The listing builds one solid part. Answer for the finished solid, in the listing's coordinates (mm). Face numbers are marked on the shaded views. Round coordinates to 2 decimals unless told otherwise and drop trailing zeros. Write each loop counter-clockwise with the first axis right and the second up, starting at its lowest first coordinate (ties: lowest second). Pieces come first, ordered by that corner, then holes. Notation, with made-up numbers: M 71.5,-16.75 L 103.5,-16.75 A14 ccw 103.5,-2.75 Z; hole C 66.25,77.25 d10. An arc over 180 degrees is marked long. Put each result on its own line as item: value. Start each with the question number.
Autodesk Fusion 360 part; units mm, degrees
sketch "Sketch1" plane through (0, 0, 0) normal (0, 0, 1) x (1, 0, 0)
  line L0 (-3, 0) -> (-6, 0)
  line L1 (-77, 52) -> (-77, 68)
  line L2 (77, 52) -> (77, 68)
  line L3 (44.954, 74) -> (71, 74)
  line L4 (44.954, 74) -> (6, 74)
  line L5 (44.954, 46) -> (6, 46)
  line L6 (44.954, 46) -> (71, 46)
  line L7 (-44.954, 74) -> (-6, 74)
  line L8 (-44.954, 46) -> (-6, 46)
  line L9 (-44.954, 74) -> (-71, 74)
  line L10 (-44.954, 46) -> (-71, 46)
  line L11 (6, 0) -> (6, 46)
  line L12 (-6, 0) -> (-6, 46)
  line L13 (-6, 120) -> (-6, 74)
  line L14 (6, 120) -> (6, 74)
  arc A0 (-71, 74) -> (-77, 68) centre (-71, 68) ccw
  arc A1 (-77, 52) -> (-71, 46) centre (-71, 52) ccw
  arc A2 (6, 120) -> (-6, 120) centre (0, 120) ccw
  arc A3 (77, 68) -> (71, 74) centre (71, 68) ccw
  arc A4 (71, 46) -> (77, 52) centre (71, 52) ccw
  arc A5 (-6, 0) -> (6, 0) centre (0, 0) ccw
  dimension "d7" = 12
  dimension "d8" = 12
  dimension "d12" = 46
extrude "Extrude1" add sketch "Sketch1" along normal blind 5
sketch "Sketch2" plane through (0, 0, 5) normal (0, 0, 1) x (-1, 0, 0)
  line L0 (71, -46) -> (6, -46)
  line L1 (6, -46) -> (6, 0)
  arc A0 (6, 0) -> (-6, 0) centre (0, 0) ccw
  line L2 (-6, 0) -> (-6, -46)
  line L3 (-6, -46) -> (-71, -46)
  arc A1 (-71, -46) -> (-77, -52) centre (-71, -52) ccw
  line L4 (-77, -52) -> (-77, -68)
  arc A2 (-77, -68) -> (-71, -74) centre (-71, -68) ccw
  line L5 (-71, -74) -> (-6, -74)
  line L6 (-6, -74) -> (-6, -120)
  arc A3 (-6, -120) -> (6, -120) centre (0, -120) ccw
  line L7 (6, -120) -> (6, -74)
  line L8 (6, -74) -> (71, -74)
  arc A4 (71, -74) -> (77, -68) centre (71, -68) ccw
  line L9 (77, -68) -> (77, -52)
  arc A5 (77, -52) -> (71, -46) centre (71, -52) ccw
  circle A6 centre (0, -120) radius 3
  circle A7 centre (0, -120) radius 1.5
  line L10 (0, 0) -> (0, -60)
  line L11 (0, -60) -> (-26, -60)
  circle A8 centre (0, 0) radius 1.5
  circle A9 centre (0, 0) radius 3
  circle A10 centre (-71, -68) radius 3
  circle A11 centre (-71, -68) radius 1.5
  circle A12 centre (-71, -52) radius 3
  circle A13 centre (-71, -52) radius 1.5
  circle A14 centre (71, -68) radius 3
  circle A15 centre (71, -68) radius 1.5
  circle A16 centre (71, -52) radius 3
  circle A17 centre (71, -52) radius 1.5
  line L12 (-6, -46) -> (6, -46)
  line L13 (-6, -74) -> (6, -74)
  line L14 (-6, -46) -> (-71, -46)
  line L15 (-77, -52) -> (-77, -68)
  line L16 (-71, -74) -> (-6, -74)
  line L17 (6, -46) -> (71, -46)
  line L18 (77, -52) -> (77, -68)
  line L19 (71, -74) -> (6, -74)
  arc A18 (77, -52) -> (71, -46) centre (71, -52) ccw
  arc A19 (71, -74) -> (77, -68) centre (71, -68) ccw
  arc A20 (-71, -46) -> (-77, -52) centre (-71, -52) ccw
  arc A21 (-77, -68) -> (-71, -74) centre (-71, -68) ccw
  arc A22 (-71, -46) -> (-77, -52) centre (-71, -52) ccw
  arc A23 (-77, -68) -> (-71, -74) centre (-71, -68) ccw
  line L20 (68, -57.5) -> (68, -62.5)
  line L21 (65.5, -65) -> (6, -65)
  line L22 (-6, -65) -> (6, -65)
  line L23 (-65.5, -65) -> (-6, -65)
  line L24 (-68, -57.5) -> (-68, -62.5)
  line L25 (-6, -55) -> (-65.5, -55)
  line L26 (-6, -55) -> (6, -55)
  line L27 (6, -55) -> (65.5, -55)
  arc A24 (-65.5, -55) -> (-68, -57.5) centre (-65.5, -57.5) ccw
  arc A25 (-68, -62.5) -> (-65.5, -65) centre (-65.5, -62.5) ccw
  arc A26 (68, -57.5) -> (65.5, -55) centre (65.5, -57.5) ccw
  arc A27 (65.5, -65) -> (68, -62.5) centre (65.5, -62.5) ccw
  dimension "d15" = 6
  dimension "d16" = 3
  dimension "d17" = 60
  dimension "d18" = 6
  dimension "d19" = 3
  dimension "d28" = 12
  dimension "d30" = 2.5
  dimension "d31" = 2.5
extrude "Extrude2" add sketch "Sketch2" along normal blind 50 contours A8 | A7 | A11 | A13 | A15 | A17
extrude "Extrude3" add sketch "Sketch2" along normal blind 40 contours A9 | A6 | A10 | A12 | A14 | A16
fillet "Fillet1" radius 2.5 4 edges at (6, 46, 2.5) (-6, 46, 2.5) (-6, 74, 2.5) (6, 74, 2.5)
fillet "Fillet2" radius 1 20 edges at (6.7322, 74.7322, 5) (6, 98.25, 5) (0, 126, 5) (-6, 98.25, 5) (-6.7322, 74.7322, 5) (-39.75, 74, 5) (-75.2426, 72.2426, 5) (-77, 60, 5) (-75.2426, 47.7574, 5) (-39.75, 46, 5) (-6.7322, 45.2678, 5) (-6, 21.75, 5) (0, -6, 5) (6, 21.75, 5) (6.7322, 45.2678, 5) (39.75, 46, 5) (75.2426, 47.7574, 5) (77, 60, 5) (75.2426, 72.2426, 5) (39.75, 74, 5)
extrude "Extrude4" cut sketch "Sketch2" against normal blind 14 contours L20 L21 L22 L23 L24 L25 L26 L27 A24 A25 A26 A27
fillet "Fillet3" radius 1 8 edges at (-68, 60, 5) (-67.2678, 64.2678, 5) (0, 65, 5) (67.2678, 64.2678, 5) (68, 60, 5) (67.2678, 55.7322, 5) (0, 55, 5) (-67.2678, 55.7322, 5)
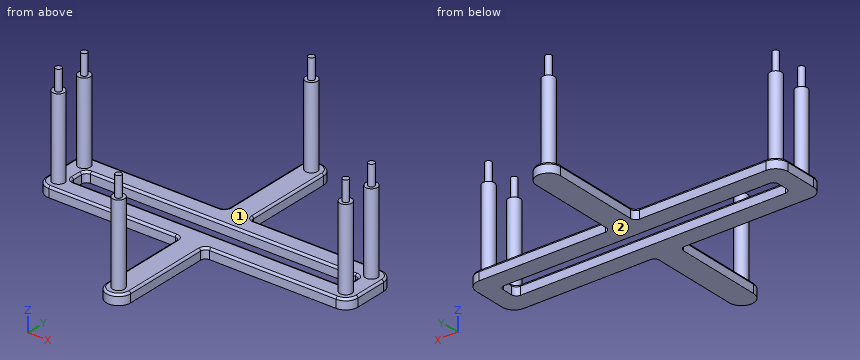
Item 1: Determine the mould class of the marked faces 1 and 2 for opening direction X: released by +X, released by -X, zero draft, split by the parting line, or undercut.
Item 2: Section B-B (y = 9) is taken. Give the vertices of the cut face in (x, z), and give its area (3 significant figures).
Item 3: Consider line 1 along Z through (x, y) = (5, 96); line 2 along Y through (x, z) = (28.5, 3.5); line 3 along X through (y, z) = (120, 16). Determine where each line is inside the solid, lowest interval first. Write a range as [from, to].
Item 4: Section A-A (z = 29) is taken. Give the vertices of the cut face in (x, y).
Item 5: Flat-ended cylindrical pins translate along their axes: pin 1 (4.5 mm diameter, centred on y = 107.5, z = 1, fed in from -X); pin 2 (1.8 mm diameter, centred on x = -1.5, y = -0.5, fed in from +Z); pin 3 (1.2 mm diameter, centred on y = 31, z = 2.5, fed in from +X); pin 4 (1.5 mm diameter, centred on y = 16.5, z = 5.5, fed in from -X). Find the tip coordinate at first contact, or state that the pin passes through.
Output values:
1. face 1: undercut
1. face 2: zero draft
2. outline: M -6,0 L 6,0 L 6,4 A1 ccw 5,5 L -5,5 A1 ccw -6,4 Z
2. area: 59.6 mm^2
3. line 1: z = [0, 5]
3. line 2: y = [46, 55], [65, 74]
3. line 3: x = [-3, 3]
4. outline: C -71,52 d6; C -71,68 d6; C 0,0 d6; C 0,120 d6; C 71,52 d6; C 71,68 d6
5. pin 1: stops at x = -6
5. pin 2: stops at z = 55
5. pin 3: stops at x = 6
5. pin 4: stops at x = -5.66
